The model under review builds one solid part; all positions refer to its coordinate system, in mm. A direction names the side the tool comes from. Coordinates: 2 decimals unless noted, no trailing zeros. Loops run counter-clockwise (first coordinate to the right, second up) from the corner with the lowest first, then second, coordinate; pieces in that order, holes last. Notation, with made-up numbers: M 24.25,88 L 28.25,88 A15 ccw 28.25,97 Z; hole C 55,-9 d7. An arc over 180 degrees is marked long. Use one line per item in the form item = value.
```python
from build123d import *

# Parameters (mm, degrees)
F0_R     = 19.12
F0_R_2   = 11.5
F1_DEPTH = 76.2
F2_R     = 19.12
F3_DEPTH = 50.8
F3_TAPER = 45
F5_DEPTH = 1
F6_COUNT = 4


with BuildPart() as f1:
    # F0 (on Top) → F1 (new body)
    with BuildSketch(Plane.XY):
        Circle(F0_R)
        Circle(F0_R_2, mode=Mode.SUBTRACT)
    extrude(amount=F1_DEPTH)

    # F2 (on face) → F3 (join)
    with BuildSketch(Plane.XY.offset(76.2)):
        Circle(F2_R)
    extrude(amount=F3_DEPTH, taper=F3_TAPER)

    # F4 (on Right) → F5 (join)
    with BuildSketch(Plane.YZ):
        Polygon((-36.5078145027, 0), (-13, 0), (-13, 26.7600230816), align=None)
    extrude(amount=F5_DEPTH)

    # F6: F1 ×4 about axis
    f6_axis = Axis((0, 0, 0), (0, 0, 1))


with BuildPart() as f1_1:
    add(f1.part)
    for i in range(1, F6_COUNT):
        add(f1.part.rotate(f6_axis, i * 360 / F6_COUNT))


solid = f1_1.part
```
1. Wall thickness on line 1 along Y through (x, z) = (0, 49); line 2 along Y through (x, z) = (2.5, 6); line 3 along X through (y, z) = (-4, 53): over which ranges is each line inside the solid? List them lowest first. Write a range as from..to.
Response values:
line_1 = -19.12..-11.5, 11.5..19.12
line_2 = -18.96..-11.22, 11.22..18.96
line_3 = -18.7..-10.78, 10.78..18.7
2. Add section C-C (y = -27.5). State the section outline as (x, z) points, then the cut area to 3 significant figures.
Response values:
outline = M 0,0 L 1,0 L 1,10.25 L 0,10.25 Z
area = 10.3 mm^2
3. The part is to be moulded in two halves that separate along Y. For faces 1 (the face through (-0.674, 5.133, 90.143)), 2 (the face through (0, 0, 76.2)), 3 (the face through (11, 6, 0)), 4 (the face through (-24, 0, 6)), say which applies: pulls with the +Y half, pulls with the -Y half, needs draft (parallel to the pull), parting line crosses it, or undercut.
Response values:
face_1 = parting line crosses it
face_2 = undercut
face_3 = needs draft
face_4 = pulls with the +Y half
4. Add section A-A (z = 74). State the section outline as (x, y) points, then the cut area to 3 significant figures.
Response values:
outline = C 0,0 d38.24; hole C 0,0 d23
area = 733 mm^2
5. Insertion check: P1, Ø3, axis at x = -13, z = 74.5, coming from the +Y side; P2, Ø14, axis at y = 27.5, z = 5.5, coming from the -X side; P3, Ø14, axis at y = -27, z = 5.5, coming from the +X side. Each pin has a flat end and moves straight along its axis. Give the tip position at first contact, or say it passes through.
Response values:
P1 = 15.27
P2 = -1
P3 = 1
6. Add section B-B (x = -22.5). State the section outline as (y, z) points, then the cut area to 3 significant figures.
Response values:
outline = M -1,0 L 0,0 L 0,15.95 L -1,15.95 Z
area = 15.9 mm^2
7. Machinability: for faces 5 (the face through (-1, 24, 6)), 6 (the face through (0, -24, 6)), 7 (the face through (24, 0, 6)), which of the approach directions +Z, -Z, +X, -X, +Y, -Y give a long, thin tool a straight path to every point of the face, cutting with its end or side? Answer none if there is none.
Response values:
face_5 = +Z, -Z, -X, +Y
face_6 = +Z, -Z, -X, -Y
face_7 = +Z, -Z, +X, -Y
